Geometry check sheet. Reference: drawing and pictorial views, mm from the part's lowest x, y, z. Give positions to 0.01 mm unless a question says otherwise; leave off trailing zeros. Order: outer loops, then holes, each group sorted by start corner. A loop starts at its lowest first (then second) coordinate and runs counter-clockwise, first axis right, second up.
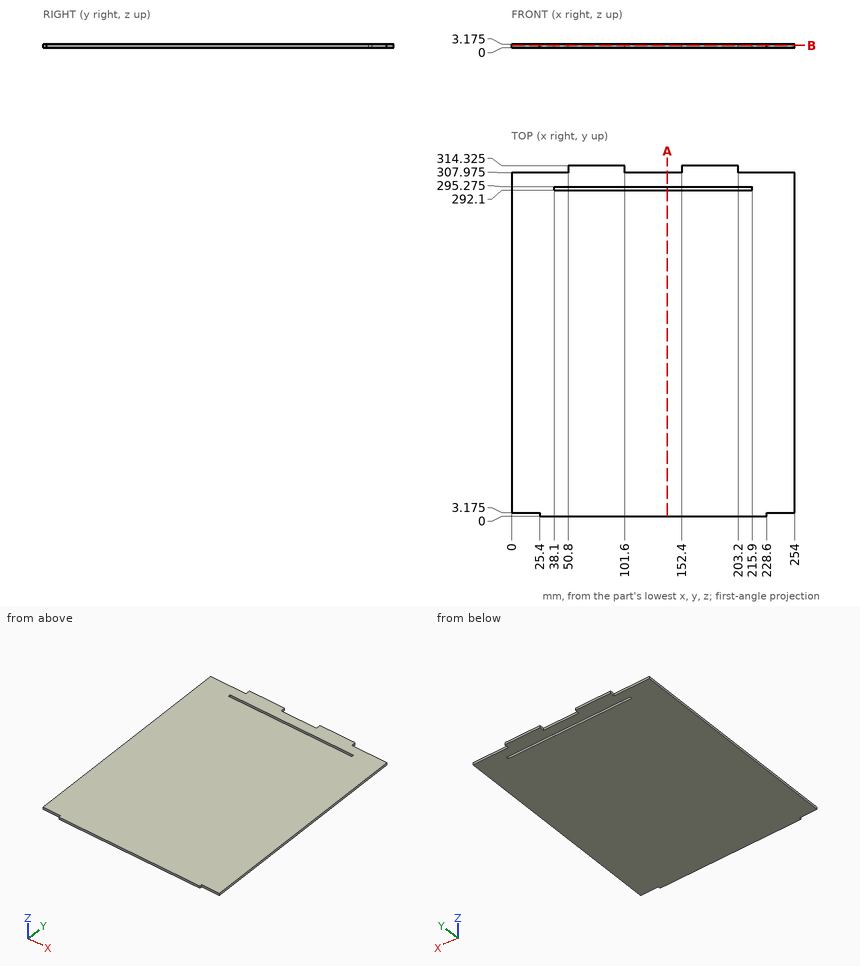
1) Material ranges on L1, parallel to Y at x = 133, z = 3 (3 decimals); L2, parallel to Y at x = 81, z = 2 (3 decimals); L3, parallel to Y at x = 220, z = 2.55 (3 decimals), recorded low to high.
Recorded:
L1: y = 0 to 292.1, 295.275 to 307.975
L2: y = 0 to 292.1, 295.275 to 314.325
L3: y = 0 to 307.975
2) Section check A-A, the plane x = 139.5. Record the cut outline in (y, z) (3 decimals), then the cut area to 3 significant figures.
Recorded:
outline: (0, 0) - (292.1, 0) - (292.1, 3.175) - (0, 3.175) - close; (295.275, 0) - (307.975, 0) - (307.975, 3.175) - (295.275, 3.175) - close
area: 968 mm2
3) Depth check by flat-ended pin: pin 1 Ø1 at (x, z) = (14, 1) entering from -Y (3 decimals); pin 2 Ø1.6 at (x, z) = (121, 1) entering from +Y (3 decimals). Enter the tip coordinate at first touch or a pass-through.
Recorded:
pin 1: stops at y = 3.175
pin 2: stops at y = 307.975
4) Section check B-B, the plane z = 2. Record the cut outline in (x, y) (3 decimals), then the cut area to 3 significant figures.
Recorded:
outline: (0, 3.175) - (25.4, 3.175) - (25.4, 0) - (228.6, 0) - (228.6, 3.175) - (254, 3.175) - (254, 307.975) - (203.2, 307.975) - (203.2, 314.325) - (152.4, 314.325) - (152.4, 307.975) - (101.6, 307.975) - (101.6, 314.325) - (50.8, 314.325) - (50.8, 307.975) - (0, 307.975) - close; hole (38.1, 292.1) - (215.9, 292.1) - (215.9, 295.275) - (38.1, 295.275) - close
area: 78,100 mm2
